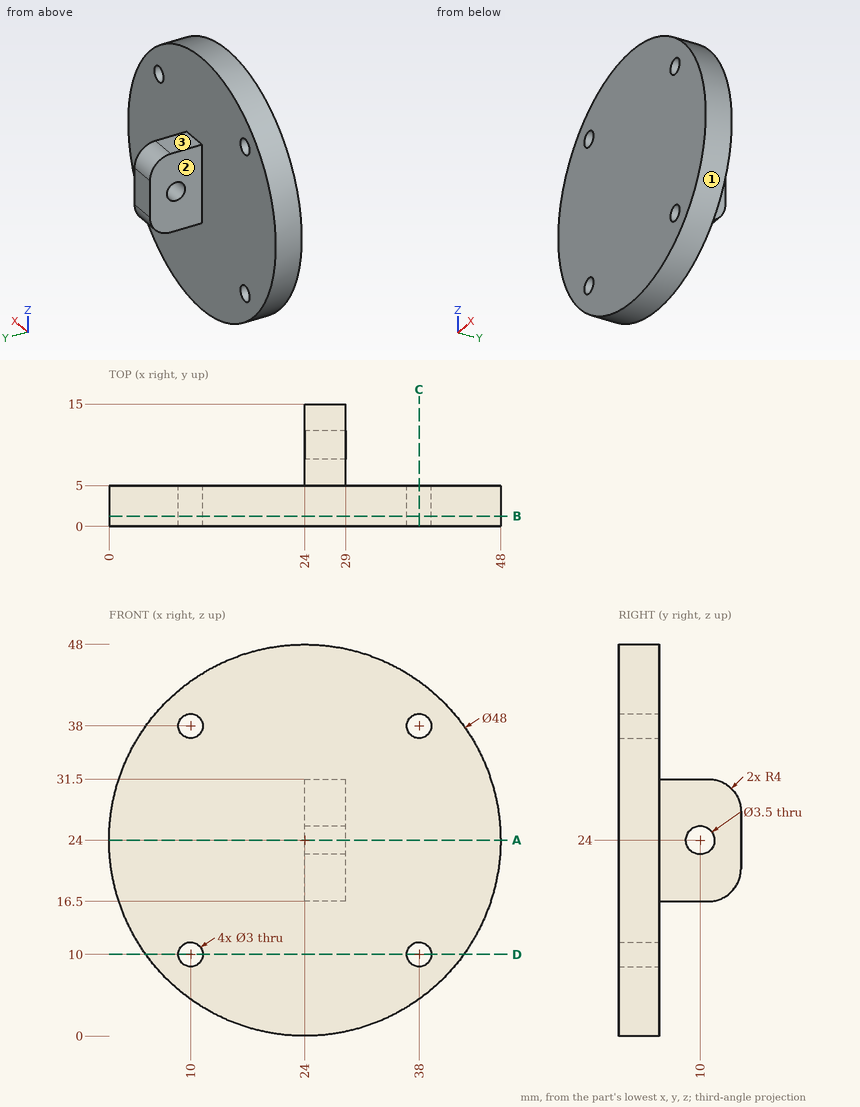
Here's the drawing with two shaded views (mm, measured from the low corner). I have some questions. A direction names the side the tool comes from. Coordinates: 2 decimals unless noted, no trailing zeros. Loops run counter-clockwise (first coordinate to the right, second up) from the corner with the lowest first, then second, coordinate; pieces in that order, holes last. Notation, with made-up numbers: M 20,16 L 78,16 A16 ccw 78,22 Z; hole C 73,-22 d3. An arc over 180 degrees is marked long. Return JSON: item names as keys, results as strings. Group by question number.
Item 1: If I drill on L1, parallel to Z at x = 38, y = 1.9; L2, parallel to X at y = 2.5, z = 37; L3, parallel to Y at x = 3, z = 20, over which ranges is the centre line in solid material (lowest first)? Write a range as from..to.
Item 2: Imagine slicing it at D-D (z = 10). Please give me the cut outline in (x, y).
Item 3: Imagine slicing it at B-B (y = 1.25). Please give me the cut outline in (x, z), and give its area (3 significant figures).
Item 4: On a 3-axis mill with a long thin cutter (end or side, diameter ignored), from which of +Z, -Z, +X, -X, +Y, -Y can I reach the whole of each face in a straight line? I mean the marked faces 1, 2 and 3. Say none if no direction works.
Item 5: Imagine slicing it at A-A (z = 24). Please give me the cut outline in (x, y), and give its area (4 significant figures).
Item 6: I'm going to push flat-ended pins straight in: pin 1 Ø4 at (x, y) = (27.5, 7.5) entering from +Z; pin 2 Ø3 at (y, z) = (8.5, 24) entering from +X; pin 3 Ø1.5 at (x, y) = (26, 9) entering from -Z; pin 4 Ø2.5 at (x, z) = (38, 10) entering from -Y. Where does each tip first touch, or does it pass through?
Item 7: Imagine slicing it at C-C (x = 38). Please give me the cut outline in (y, z).
Verdict:
{
 "1": {"L1": "z = 4.51..8.5, 11.5..36.5, 39.5..43.49", "L2": "x = 3.83..8.88, 11.12..36.88, 39.12..44.17", "L3": "y = 0..5"},
 "2": {"outline": "M 4.51,0 L 8.5,0 L 8.5,5 L 4.51,5 Z; M 11.5,0 L 36.5,0 L 36.5,5 L 11.5,5 Z; M 39.5,0 L 43.49,0 L 43.49,5 L 39.5,5 Z"},
 "3": {"outline": "C 24,24 d48; hole C 10,10 d3; hole C 10,38 d3; hole C 38,10 d3; hole C 38,38 d3", "area": "1,780 mm^2"},
 "4": {"face 1": "+Y, -Y", "face 2": "+Z, -Z, -X, +Y", "face 3": "+Z, +X, -X, +Y"},
 "5": {"outline": "M 0,0 L 48,0 L 48,5 L 29,5 L 29,8.25 L 24,8.25 L 24,5 L 0,5 Z; M 24,11.75 L 29,11.75 L 29,15 L 24,15 Z", "area": "272.5 mm^2"},
 "6": {"pin 1": "stops at z = 31.5", "pin 2": "stops at x = 29", "pin 3": "stops at z = 16.5", "pin 4": "passes through"},
 "7": {"outline": "M 0,4.51 L 5,4.51 L 5,8.5 L 0,8.5 Z; M 0,11.5 L 5,11.5 L 5,36.5 L 0,36.5 Z; M 0,39.5 L 5,39.5 L 5,43.49 L 0,43.49 Z"}
}
